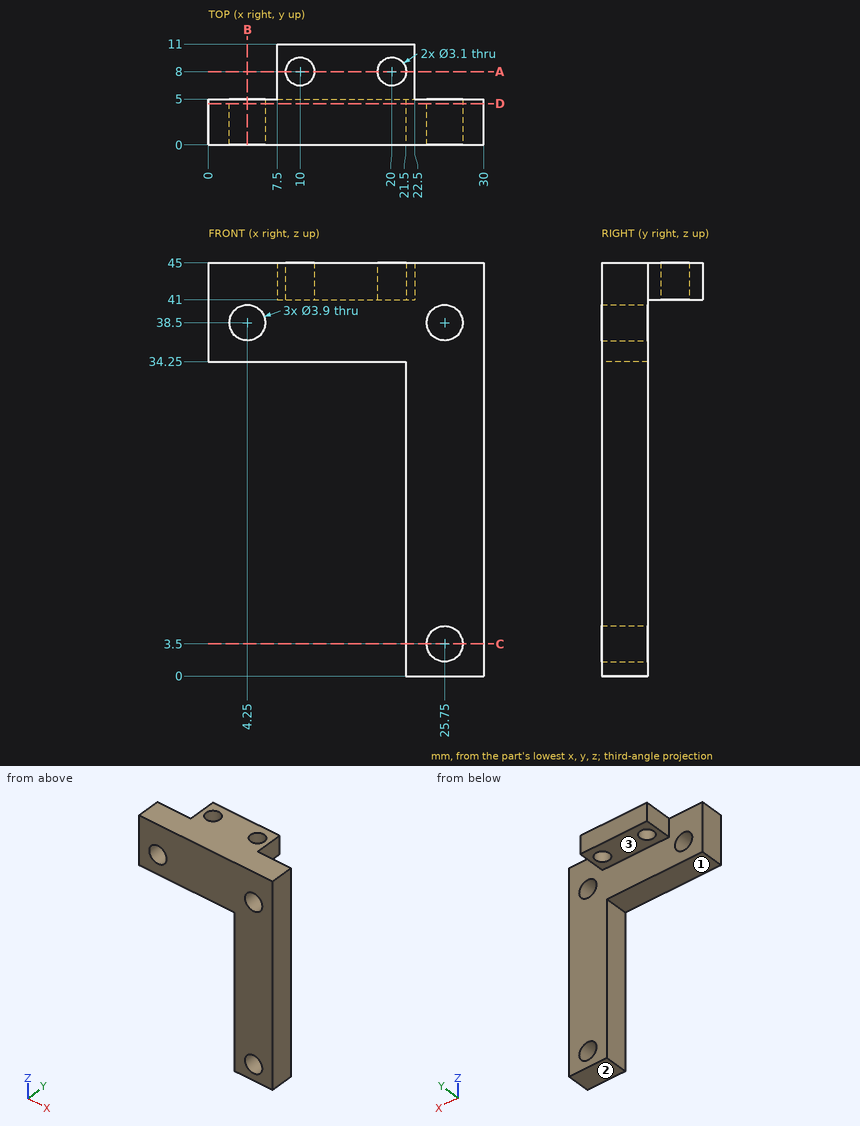
Job drawing, mm, ordinate dimensions from the low corner. One solid piece. A direction names the side the tool comes from. Round coordinates to 2 decimals unless told otherwise and drop trailing zeros. Order: outer loops, then holes, each group sorted by start corner. A loop starts at its lowest first (then second) coordinate and runs counter-clockwise, first axis right, second up. Notation, with made-up numbers: M 4.25,-29.75 L 25.25,-29.75 A24 ccw 25.25,5.25 Z; hole C 30.25,41 d3. An arc over 180 degrees is marked long. Write each question's results on one line, items separated by ' | '. Start each with the question number.
(1) Saw through at B-B, the plane x = 4.25. Give the cut face in (y, z).
(2) Saw through at D-D, the plane y = 4.5. Give the cut face in (x, z), then the cut area to 3 significant figures.
(3) Probe probe 1 along X at (y, z) = (1.7, 38.5); probe 2 along Z at (x, y) = (25.75, 1.5); probe 3 along Y at (x, z) = (20, 44.1). List the from-to ranges inside material, lowest first. Write a range as from..to.
(4) Saw through at C-C, the plane z = 3.5. Give the cut face in (x, y).
(5) Drop flat-ended pins along their axis: pin 1 (1.2 mm diameter, centred on y = 8, z = 43.5, fed in from +X); pin 2 (1.8 mm diameter, centred on x = 14, y = 9, fed in from -Z); pin 3 (1 mm diameter, centred on x = 24.5, z = 6.5, fed in from +Y); pin 4 (2 mm diameter, centred on x = 5.5, y = 9, fed in from -Z). Give the stop position or say it passes through.
(6) Saw through at A-A, the plane y = 8. Give the cut face in (x, z), then the cut area to 3 significant figures.
(7) Which spindle directions (+Z, -Z, +X, -X, +Y, -Y) get a long thin tool onto all of the face, cutting with end or side? Do the marked faces 1, 2 and 3. Say none if no direction does.
Established:
1) outline: M 0,34.25 L 5,34.25 L 5,36.55 L 0,36.55 Z; M 0,40.45 L 5,40.45 L 5,45 L 0,45 Z
2) outline: M 0,34.25 L 21.5,34.25 L 21.5,0 L 30,0 L 30,45 L 0,45 Z; hole C 4.25,38.5 d3.9; hole C 25.75,3.5 d3.9; hole C 25.75,38.5 d3.9 | area: 578 mm^2
3) probe 1: x = 0..2.3, 6.2..23.8, 27.7..30 | probe 2: z = 0..1.55, 5.45..36.55, 40.45..45 | probe 3: y = 0..6.45, 9.55..11
4) outline: M 21.5,0 L 23.8,0 L 23.8,5 L 21.5,5 Z; M 27.7,0 L 30,0 L 30,5 L 27.7,5 Z
5) pin 1: stops at x = 22.5 | pin 2: stops at z = 41 | pin 3: stops at y = 5 | pin 4: passes through
6) outline: M 7.5,41 L 8.45,41 L 8.45,45 L 7.5,45 Z; M 11.55,41 L 18.45,41 L 18.45,45 L 11.55,45 Z; M 21.55,41 L 22.5,41 L 22.5,45 L 21.55,45 Z | area: 35.2 mm^2
7) face 1: -Z, -X, +Y, -Y | face 2: -Z, +X, -X, +Y, -Y | face 3: -Z, +X, -X, +Y
